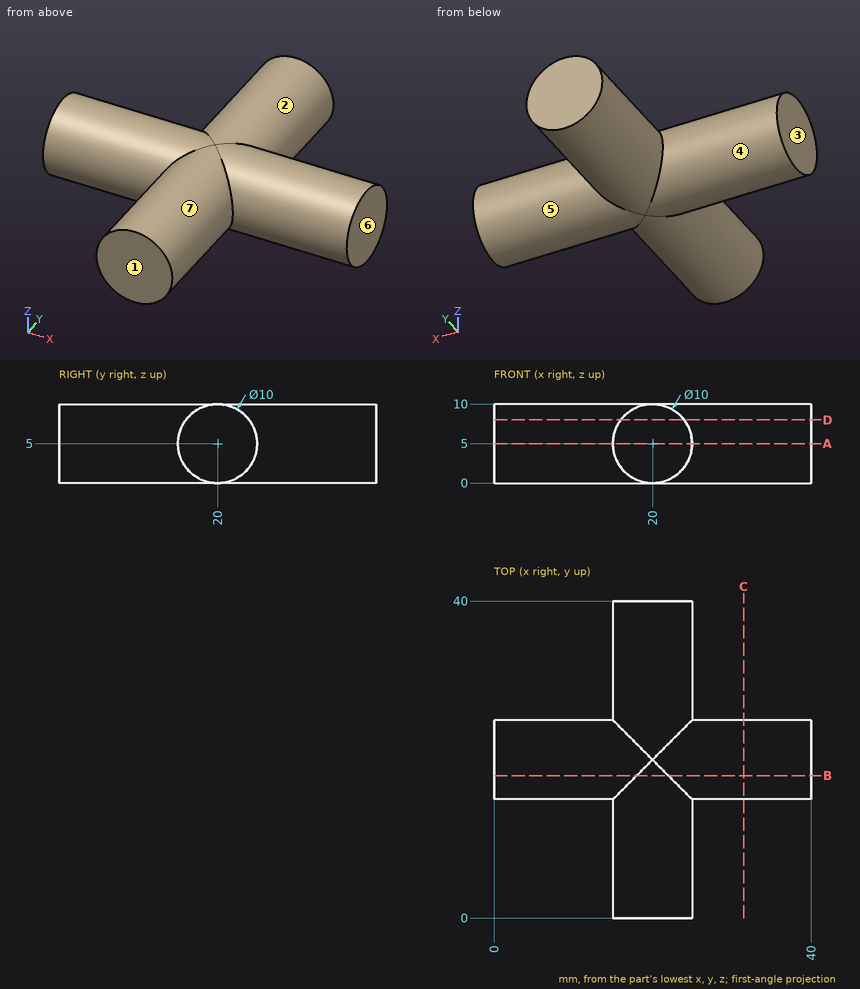
Drawing for the job (mm, zero at the part's lowest x, y, z). A direction names the side the tool comes from. Round coordinates to 2 decimals unless told otherwise and drop trailing zeros. Loops run counter-clockwise (first coordinate to the right, second up) from the corner with the lowest first, then second, coordinate; pieces in that order, holes last. Notation, with made-up numbers: (63, 51.25) - (106, 51.25) arc R12 ccw to (106, 60.25) - close; hole circle Ø1 at (44, 4). An arc over 180 degrees is marked (long way). Return JSON: item names as keys, results as strings. Group by question number.
Q1. Band-saw the part on B-B on y = 18. Give the cut face in (x, z).
Q2. Band-saw the part on D-D on z = 8. Give the cut face in (x, y).
Q3. Drill centre lines: line 1 along X through (y, z) = (2.5, 4.75); line 2 along Y through (x, z) = (31, 5); line 3 along Z through (x, y) = (18, 28). Where is each one in solid material? Low to high. Write a range as [from, to].
Q4. Band-saw the part on C-C on x = 31.5. Give the cut face in (y, z).
Q5. Tool access for the marked faces 1, 2, 3, 4 and 5: list every direction of +Z, -Z, +X, -X, +Y, -Y with a clear straight run to the whole face (end or side of a thin tool).
Q6. Band-saw the part on A-A on z = 5. Give the cut face in (x, y).
Q7. Two-plate mould, pull along Z, no slides. Class the marked faces 6 and 7: +Z half, -Z half, draft (parallel to the pull), parting line (faces both ways), or undercut.
Q8. Flat gauge pins, fed straight in: pin 1 Ø10 at (x, y) = (30, 12) entering from -Z; pin 2 Ø6 at (y, z) = (9, 7.5) entering from -X; pin 3 Ø3 at (x, z) = (31, 3) entering from +Y. Where does each tip first touch, or does it go through?
Solutions:
{
 "1": {"outline": "(0, 0.42) - (18, 0.42) arc R5 ccw to (22, 0.42) - (40, 0.42) - (40, 9.58) - (22, 9.58) arc R5 ccw to (18, 9.58) - (0, 9.58) - close"},
 "2": {"outline": "(0, 16) - (16, 16) - (16, 0) - (24, 0) - (24, 16) - (40, 16) - (40, 24) - (24, 24) - (24, 40) - (16, 40) - (16, 24) - (0, 24) - close"},
 "3": {"line 1": "x = [15.01, 24.99]", "line 2": "y = [15, 25]", "line 3": "z = [0.42, 9.58]"},
 "4": {"outline": "circle Ø10 at (20, 5)"},
 "5": {"face 1": "+Z, -Z, +X, -X, -Y", "face 2": "+Y", "face 3": "+Z, -Z, -X, +Y, -Y", "face 4": "-X", "face 5": "+X"},
 "6": {"outline": "(0, 15) - (15, 15) - (15, 0) - (25, 0) - (25, 15) - (40, 15) - (40, 25) - (25, 25) - (25, 40) - (15, 40) - (15, 25) - (0, 25) - close"},
 "7": {"face 6": "draft", "face 7": "parting line"},
 "8": {"pin 1": "stops at z = 1", "pin 2": "stops at x = 15", "pin 3": "stops at y = 24.97"}
}
